Source: CAD feature listing. Evaluate the final solid. Frame: model axes, mm. Round coordinates to 2 decimals unless told otherwise and drop trailing zeros. Loops run counter-clockwise (first coordinate to the right, second up) from the corner with the lowest first, then second, coordinate; pieces in that order, holes last. Notation, with made-up numbers: (63.5, 55.5) -> (70.5, 55.5) arc R18 ccw to (70.5, 60.5) -> close; hole circle Ø2 at (75.25, -30). An arc over 180 degrees is marked (long way). Put each result on its own line as item: value. Start each with the question number.
1. Cut plane C-C (y = 6.75). Return the cut outline in (x, z) (1 decimal).
2. Cut plane A-A (z = -11). Return the cut outline in (x, y) (1 decimal), then the cut area to 3 significant figures.
3. Cut plane B-B (x = -6.75). Return the cut outline in (y, z) (1 decimal), then the cut area to 3 significant figures.
4. Draft query along X for faces 1 (the cylindrical face through (-19, 0.5, -9.6)), 2 (the cylindrical face through (-11.285, 6.517, -2.649)), 3 (the flat face through (0, 6, -10)). Return one class per face: pulls with the +X half, pulls with the -X half, needs draft (parallel to the pull), parting line crosses it, or undercut.
5. Material intervals for L1, parallel to Z at x = -12.5, y = 6; L2, parallel to Z at x = -10.75, y = 4; L3, parallel to X at y = 1.25, z = -12.75, sorted ascending.
Autodesk Inventor part; units mm, degrees
ref_plane "Work Plane2" through (-19.431, 0, -9.7155) normal (0, 0, 1) x (1, 0, 0)
ref_plane "YZ Plane" through (0, 0, 0) normal (1, 0, 0) x (0, 1, 0)
ref_plane "XZ Plane" through (0, 0, 0) normal (0, 1, 0) x (-1, 0, 0)
sketch "Sketch1" plane through (0, 0, 0) normal (0, 1, 0) x (-1, 0, 0)
  line L0 (0, 0) -> (19.431, 0)
  line L1 (19.431, 0) -> (19.431, -19.431)
  line L2 (19.431, -19.431) -> (0, -19.431)
  line L3 (0, -19.431) -> (0, 0)
  dimension "d0" = 19.431
  dimension "d1" = 19.431
extrude "Extrusion1" add sketch "Sketch1" along normal blind 10.922
ref_plane "Work Plane2" through (-19.431, 0, -9.7155) normal (0, 0, 1) x (1, 0, 0)
sketch "Sketch2" plane through (-19.431, 0, -9.7155) normal (0, 0, 1) x (1, 0, 0)
  arc A0 (9.7155, -5.2517) -> (16.9545, 1.9873) centre (9.7155, 1.9873) ccw
  line L0 (16.9545, 1.9873) -> (16.9545, 10.922)
  line L1 (19.431, 10.922) -> (0, 10.922)
  line L2 (9.7155, -5.3792) -> (9.7155, 10.922)
  line L3 (16.9545, 10.922) -> (9.7155, 10.922)
  point P0 (19.431, 0)
  dimension "d4" = 14.478
revolve "Revolution1" cut sketch "Sketch2" angle 360 about axis through (-9.7155, -5.3792, -9.7155) along (0, 1, 0)
fillet "Fillet1" radius 1.5875 2 edges at (-9.7155, 0, -19.431) (0, 0, -9.7155)
fillet "Fillet2" radius 1.5875 9 edges at (-19.431, 0, -8.9218) (-19.431, 0.465, -18.966) (-19.431, 6.2548, -19.431) (-0.465, 0.465, 0) (0, 6.2548, 0) (-10.5092, 0, 0) (-0.465, 0.465, -18.966) (0, 6.2548, -19.431) (-19.431, 5.461, 0)
equation "\"d1\" = d0"
properties part number "tail-rolley-polley"
Solution:
1. outline: (-19.4, -17.8) arc R1.6 ccw to (-17.8, -19.4) -> (-1.6, -19.4) arc R1.6 ccw to (0, -17.8) -> (0, -1.6) arc R1.6 ccw to (-1.6, 0) -> (-17.8, 0) arc R1.6 ccw to (-19.4, -1.6) -> close; hole circle Ø14.5 at (-9.7, -9.7)
2. outline: (-19.4, 1.6) arc R1.6 ccw to (-17.8, 0) -> (-16.6, 0) arc R7.1 cw to (-16.8, 2) -> (-16.8, 10.9) -> (-19.4, 10.9) -> close; (-2.9, 0) -> (-1.6, 0) arc R1.6 ccw to (0, 1.6) -> (0, 10.9) -> (-2.6, 10.9) -> (-2.6, 2) arc R7.1 cw to start
2. area: 55.9 mm^2
3. outline: (0, -17.8) arc R1.6 ccw to (1.6, -19.4) -> (10.9, -19.4) -> (10.9, -16.3) -> (2, -16.3) arc R6.6 cw to (0, -16) -> close; (0, -3.4) arc R6.6 cw to (2, -3.1) -> (10.9, -3.1) -> (10.9, 0) -> (1.6, 0) arc R1.6 ccw to (0, -1.6) -> close
3. area: 67.3 mm^2
4. face 1: pulls with the -X half
4. face 2: undercut
4. face 3: pulls with the +X half
5. L1: z = -19.43 to -16.4, -3.03 to 0
5. L2: z = -19.43 to -16.88, -2.55 to 0
5. L3: x = -19.39 to -16.25, -3.18 to -0.04
